Geometry check sheet. Reference: the model listing, model coordinates, mm. Give positions to 0.01 mm unless a question says otherwise; leave off trailing zeros. Order: outer loops, then holes, each group sorted by start corner. A loop starts at its lowest first (then second) coordinate and runs counter-clockwise, first axis right, second up.
Autodesk Fusion 360 part; units mm, degrees
sketch "スケッチ17" plane through (0, 0, 0) normal (0, 0, 1) x (1, 0, 0)
  circle A0 centre (0, 0) radius 2.5
  dimension "d50" = 5
extrude "押し出し14" add sketch "スケッチ17" along normal blind 3.8
sketch "スケッチ18" plane through (0, 0, 3.8) normal (0, 0, 1) x (-1, 0, 0)
  circle A0 centre (0, 0) radius 2.5
  circle A1 centre (0, 0) radius 2.25
  dimension "d53" = 4.5
extrude "押し出し15" add sketch "スケッチ18" along normal blind 16.4 contours A1
sketch "スケッチ19" plane through (0, 0, 20.2) normal (0, 0, 1) x (-1, 0, 0)
  circle A0 centre (0, 0) radius 2.25
  circle A1 centre (0, 0) radius 2.5
  dimension "d56" = 5
extrude "押し出し16" add sketch "スケッチ19" along normal blind 3.8 contours A0 | A1
sketch "スケッチ20" plane through (0, 0, 24) normal (0, 0, 1) x (-1, 0, 0)
  circle A0 centre (0, 0) radius 2.5
  circle A1 centre (0, 0) radius 1.585
  dimension "d59" = 3.17
extrude "押し出し17" cut sketch "スケッチ20" against normal blind 24 contours A1
Item 1: Sectioned sample at C-C (z = 16). Enter the section's corners in (x, y) (3 decimals), and give its area (3 significant figures).
Reported:
outline: circle Ø4.5 at (0, 0); hole circle Ø3.17 at (0, 0)
area: 8.01 mm2
Item 2: Sectioned sample at D-D (z = 3). Enter the section's corners in (x, y) (3 decimals), and give its area (3 significant figures).
Reported:
outline: circle Ø5 at (0, 0); hole circle Ø3.17 at (0, 0)
area: 11.7 mm2
Item 3: Scan lines: L1, parallel to Z at x = 1.1, y = -2; L2, parallel to Y at x = 0, z = 16.25 (3 decimals). Record each from-to range of solid material in increasing order.
Reported:
L1: z = 0 to 3.8, 20.2 to 24
L2: y = -2.25 to -1.585, 1.585 to 2.25
Item 4: Draft check along X on faces 1 (the cylindrical face through (0.29, 2.23, 11.89)), 2 (the flat face through (-2, 0, 24)), 3 (the cylindrical face through (1.26, 0.96, 12.17)). Enter one of: released by +X, released by -X, zero draft, split by the parting line, or undercut.
Reported:
face 1: split by the parting line
face 2: zero draft
face 3: undercut
Item 5: Gauge pin test, flat ends, axial feed: pin 1 (3 mm diameter, centred on x = 0, y = 0, fed in from +Z); pin 2 (3 mm diameter, centred on y = 0.5, z = 17.5, fed in from +X). Record the tip position at first contact, or that the pin passes through.
Reported:
pin 1: passes through
pin 2: stops at x = 2.25
Item 6: Sectioned sample at A-A (y = 0). Enter the section's corners in (x, z) (3 decimals), and give its area (3 significant figures).
Reported:
outline: (-2.5, 0) - (-1.585, 0) - (-1.585, 24) - (-2.5, 24) - (-2.5, 20.2) - (-2.25, 20.2) - (-2.25, 3.8) - (-2.5, 3.8) - close; (1.585, 0) - (2.5, 0) - (2.5, 3.8) - (2.25, 3.8) - (2.25, 20.2) - (2.5, 20.2) - (2.5, 24) - (1.585, 24) - close
area: 35.7 mm2
